from build123d import *

# Parameters (mm, degrees)
F0_W     = 214
F0_H     = 5
F0_W_2   = 202
F0_W_3   = 10
F0_H_2   = 6
F0_W_4   = 6
F1_DEPTH = 10
F2_DEPTH = 162
F3_DEPTH = 6
F4_R     = 3.25
F4_R_2   = 3
F5_DEPTH = 25


with BuildPart() as f1:
    # F0 (on Top) → F1 (new body)
    with BuildSketch(Plane.XY):
        Polygon((107, 3), (-107, 3), (-107, -3), (-101, -3), (101, -3), (107, -3), align=None)
        with Locations((0, 5.5)):
            Rectangle(F0_W, F0_H)
        with Locations((0, -5.5)):
            Rectangle(F0_W_2, F0_H)
        with Locations((-112, 0)):
            Rectangle(F0_W_3, F0_H_2)
        with Locations((-112, 5.5)):
            Rectangle(F0_W_3, F0_H)
        with Locations((-112, -5.5)):
            Rectangle(F0_W_3, F0_H)
        with Locations((-104, -5.5)):
            Rectangle(F0_W_4, F0_H)
        with Locations((112, 0)):
            Rectangle(F0_W_3, F0_H_2)
        with Locations((112, 5.5)):
            Rectangle(F0_W_3, F0_H)
        with Locations((104, -5.5)):
            Rectangle(F0_W_4, F0_H)
        with Locations((112, -5.5)):
            Rectangle(F0_W_3, F0_H)
    extrude(amount=-F1_DEPTH)

    # F0 (on Top) → F2 (join)
    with BuildSketch(Plane.XY):
        with Locations((0, 5.5)):
            Rectangle(F0_W, F0_H)
        with Locations((-112, 5.5)):
            Rectangle(F0_W_3, F0_H)
        with Locations((-112, 0)):
            Rectangle(F0_W_3, F0_H_2)
        with Locations((-112, -5.5)):
            Rectangle(F0_W_3, F0_H)
        with Locations((112, 5.5)):
            Rectangle(F0_W_3, F0_H)
        with Locations((112, 0)):
            Rectangle(F0_W_3, F0_H_2)
        with Locations((112, -5.5)):
            Rectangle(F0_W_3, F0_H)
        with Locations((104, -5.5)):
            Rectangle(F0_W_4, F0_H)
        with Locations((-104, -5.5)):
            Rectangle(F0_W_4, F0_H)
    extrude(amount=F2_DEPTH)

    # F0 (on Top) → F3 (join)
    with BuildSketch(Plane.XY):
        with Locations((0, -5.5)):
            Rectangle(F0_W_2, F0_H)
    extrude(amount=F3_DEPTH)

    # F4 (on face) → F5 (cut)
    with BuildSketch(Plane.XZ.offset(-3)):
        with Locations((0, 115)):
            Circle(F4_R)
        with Locations((72, 156)):
            Circle(F4_R_2)
        with Locations((0, 35)):
            Circle(F4_R)
        with Locations((-72, 156)):
            Circle(F4_R_2)
    extrude(amount=-F5_DEPTH, mode=Mode.SUBTRACT)


solid = f1.part
The listing builds one solid part. Answer for the finished solid, in the listing's coordinates (mm). A direction names the side the tool comes from. Coordinates: 2 decimals unless noted, no trailing zeros. Order: outer loops, then holes, each group sorted by start corner. A loop starts at its lowest first (then second) coordinate and runs counter-clockwise, first axis right, second up.
Q1. Given P1, Ø10.5, axis at x = 0, z = 35, coming from the -Y side; P2, Ø4, axis at x = -21.5, y = -4.5, coming from the +Z side, each flat-ended and moving along its own axis, determine where each tip first touches the part or whether it passes through.
Q2. Consider line 1 (Z direction, x = 0, y = 4.1); line 2 (X direction, y = 6.95, z = 156); line 3 (X direction, y = -1.75, z = 8). Determine where each line is inside the solid, lowest interval first.
Q3. A cutting plane is placed at D-D, the plane z = 29. Write down the section's boundary in (x, y).
Q4. A cutting plane is placed at B-B, the plane x = 0. Write down the section's boundary in (y, z), and give its area (3 significant figures).
Q5. Which of the six approach directions +Z, -Z, +X, -X, +Y, -Y give full straight-line access (tool end or side, diameter ignored) to faces 4 (the face through (-0.5, -8, 5.5)), 5 (the face through (107, 0, 80)), 6 (the face through (-1, -5, 6))?
Q6. A cutting plane is placed at A-A, the plane z = 156. Write down the section's boundary in (x, y).
Q7. A cutting plane is placed at C-C, the plane x = 89.5. Write down the section's boundary in (y, z).
Q8. For a pull along X with two mould halves and no side action, classify faces 1 (the face through (-0.705, 5.465, 31.827)), 2 (the face through (-117, 0, 75)), 3 (the face through (-2, 0, -10)) as pulls with the +X half, pulls with the -X half, needs draft (parallel to the pull), parting line crosses it, or undercut.
Answers follow:
1. P1: stops at y = 3
1. P2: stops at z = 6
2. line 1: z = -10 to 31.75, 38.25 to 111.75, 118.25 to 162
2. line 2: x = -117 to -75, -69 to 69, 75 to 117
2. line 3: x = -117 to -107, 107 to 117
3. outline: (-117, -8) - (-101, -8) - (-101, -3) - (-107, -3) - (-107, 3) - (107, 3) - (107, -3) - (101, -3) - (101, -8) - (117, -8) - (117, 8) - (-117, 8) - close
4. outline: (-8, -10) - (8, -10) - (8, 31.75) - (3, 31.75) - (3, 0) - (-3, 0) - (-3, 6) - (-8, 6) - close; (3, 38.25) - (8, 38.25) - (8, 111.75) - (3, 111.75) - close; (3, 118.25) - (8, 118.25) - (8, 162) - (3, 162) - close
4. area: 935 mm2
5. face 4: +Z, -Z, +X, -X, -Y
5. face 5: +Z
5. face 6: +Z, -Y
6. outline: (-117, -8) - (-101, -8) - (-101, -3) - (-107, -3) - (-107, 3) - (-75, 3) - (-75, 8) - (-117, 8) - close; (-69, 3) - (69, 3) - (69, 8) - (-69, 8) - close; (75, 3) - (107, 3) - (107, -3) - (101, -3) - (101, -8) - (117, -8) - (117, 8) - (75, 8) - close
7. outline: (-8, -10) - (8, -10) - (8, 162) - (3, 162) - (3, 0) - (-3, 0) - (-3, 6) - (-8, 6) - close
8. face 1: undercut
8. face 2: pulls with the -X half
8. face 3: needs draft
